Work out the finished part from the listing and answer in its coordinate system (mm). Face numbers are marked on the shaded views. A direction names the side the tool comes from. Give positions to 0.01 mm unless a question says otherwise; leave off trailing zeros. Write each loop counter-clockwise with the first axis right and the second up, starting at its lowest first coordinate (ties: lowest second). Pieces come first, ordered by that corner, then holes.
1) Find section D-D (x = 37.5). Determine the outline of the cut face in (y, z).
2) A tool of negligible diameter and unlimited length cuts with its end or side. For the marked faces 1, 2 and 3, from which of +Z, -Z, +X, -X, +Y, -Y can it reach the whole face along a straight path? Write none if from no direction.
3) Given pin 1 Ø3 at (y, z) = (14, 3.5) entering from +X; pin 2 Ø1.3 at (x, z) = (67.5, 0.5) entering from +Y; pin 3 Ø10 at (x, y) = (15.5, 8) entering from -Z; pin 4 Ø2 at (x, y) = (19.5, 2.5) entering from +Z, each flat-ended and moving along its own axis, determine where each tip first touches the part or whether it passes through.
4) Find section C-C (z = 4). Determine the outline of the cut face in (x, y), plus the area to 3 significant figures.
5) Find section A-A (x = 26.45). Determine the outline of the cut face in (y, z), plus the area to 3 significant figures.
6) Find section B-B (y = 12.5). Determine the outline of the cut face in (x, z), plus the area to 3 significant figures.
7) Straight lines are drawn through the part: probe 1 along X at (y, z) = (11.25, 1.5); probe 2 along Y at (x, z) = (26.45, 0.5); probe 3 along X at (y, z) = (12.75, 0.75). For each, find the intervals that lie inside material, in ascending order.
```python
from build123d import *

# Parameters (mm, degrees)
ESQUISSE1_R        = 1.75
BOSS_EXTRU_1_DEPTH = 1.6
ESQUISSE2_W        = 20
ESQUISSE2_H        = 7.3
BOSS_EXTRU_2_DEPTH = 6.2


with BuildPart() as part:
    # Esquisse1 → Boss.-Extru.1 (new body)
    with BuildSketch(Plane.XY):
        with BuildLine():
            Line((4.6, 0), (73.4, 0))
            ThreePointArc((73.4, 0), (76.652691193, 1.347308807), (78, 4.6))
            Line((78, 4.6), (78, 4.7))
            ThreePointArc((78, 4.7), (76.652691193, 7.952691193), (73.4, 9.3))
            Line((73.4, 9.3), (61.92, 9.3))
            ThreePointArc((61.92, 9.3), (55.966160902, 11.766160902), (53.5, 17.72))
            Line((53.5, 17.72), (24.5, 17.72))
            ThreePointArc((24.5, 17.72), (22.033839098, 11.766160902), (16.08, 9.3))
            Line((16.08, 9.3), (4.6, 9.3))
            ThreePointArc((4.6, 9.3), (1.347308807, 7.952691193), (0, 4.7))
            Line((0, 4.7), (0, 4.6))
            ThreePointArc((0, 4.6), (1.347308807, 1.347308807), (4.6, 0))
        make_face()
        with Locations((26.45, 11.72)):
            Circle(ESQUISSE1_R, mode=Mode.SUBTRACT)
        with Locations(Location((51.55, 11.72, 0), (0, 0, 180))):
            Circle(ESQUISSE1_R, mode=Mode.SUBTRACT)
    extrude(amount=BOSS_EXTRU_1_DEPTH)

    # Esquisse2 → Boss.-Extru.2 (add)
    with BuildSketch(Plane.XY.offset(1.6)):
        with Locations((39, 14.07)):
            Rectangle(ESQUISSE2_W, ESQUISSE2_H)
    extrude(amount=BOSS_EXTRU_2_DEPTH)


solid = part.part
```
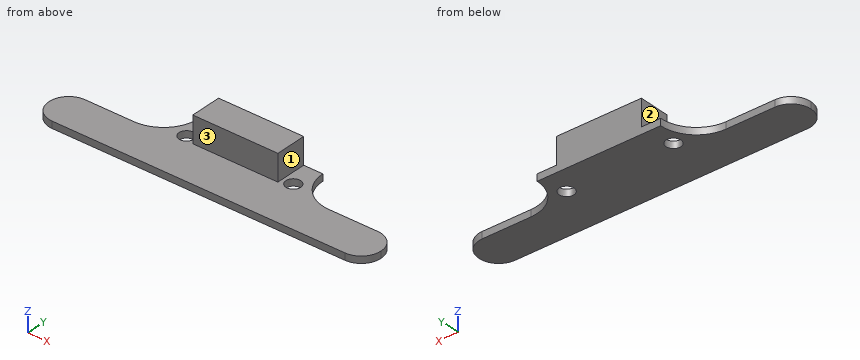
Results:
1. outline: (0, 0) - (17.72, 0) - (17.72, 7.8) - (10.42, 7.8) - (10.42, 1.6) - (0, 1.6) - close
2. face 1: +Z, +X, +Y, -Y
2. face 2: +Z, -X, +Y, -Y
2. face 3: +Z, +X, -X, -Y
3. pin 1: stops at x = 49
3. pin 2: stops at y = 9.3
3. pin 3: stops at z = 0
3. pin 4: stops at z = 1.6
4. outline: (29, 10.42) - (49, 10.42) - (49, 17.72) - (29, 17.72) - close
4. area: 146 mm2
5. outline: (0, 0) - (9.97, 0) - (9.97, 1.6) - (0, 1.6) - close; (13.47, 0) - (17.72, 0) - (17.72, 1.6) - (13.47, 1.6) - close
5. area: 22.8 mm2
6. outline: (22.69, 0) - (24.88, 0) - (24.88, 1.6) - (22.69, 1.6) - close; (28.02, 0) - (49.98, 0) - (49.98, 1.6) - (49, 1.6) - (49, 7.8) - (29, 7.8) - (29, 1.6) - (28.02, 1.6) - close; (53.12, 0) - (55.31, 0) - (55.31, 1.6) - (53.12, 1.6) - close
6. area: 166 mm2
7. probe 1: x = 21.47 to 24.76, 28.14 to 49.86, 53.24 to 56.53
7. probe 2: y = 0 to 9.97, 13.47 to 17.72
7. probe 3: x = 22.88 to 25.04, 27.86 to 50.14, 52.96 to 55.12
